For this review, use the dimensioned drawing (mm, ordinates from the lowest corner) and the shaded views. Round coordinates to 2 decimals unless told otherwise and drop trailing zeros. Write each loop counter-clockwise with the first axis right and the second up, starting at its lowest first coordinate (ties: lowest second). Pieces come first, ordered by that corner, then holes. Notation, with made-up numbers: M -18,73 L 29,73 A16 ccw 29,85 Z; hole C 61.25,-37.5 d5. An arc over 180 degrees is marked long. Use one line per item in the form item = value. Start each with the question number.
Item 1: Add section B-B (z = 16.75). State the section outline as (x, y) points, and give its area (3 significant figures).
Item 2: Add section A-A (x = 71). State the section outline as (y, z) points, and give its area (3 significant figures).
Item 3: For line 1 (Y direction, x = 20, z = 11); line 2 (X direction, y = 615, z = 21.5); line 3 (Y direction, x = 26, z = 9.5), list the stretches that pass through material, from the lowest coordinate up. Write a range as [from, to].
Item 4: For P1, Ø8, axis at x = 49.5, z = 4, coming from the -Y side; P2, Ø3, axis at x = 64, z = 12, coming from the -Y side; P3, Ø2, axis at x = 8, z = 8, coming from the -Y side, all flat-tipped, find the tip position at first contact; note any pin that passes through.
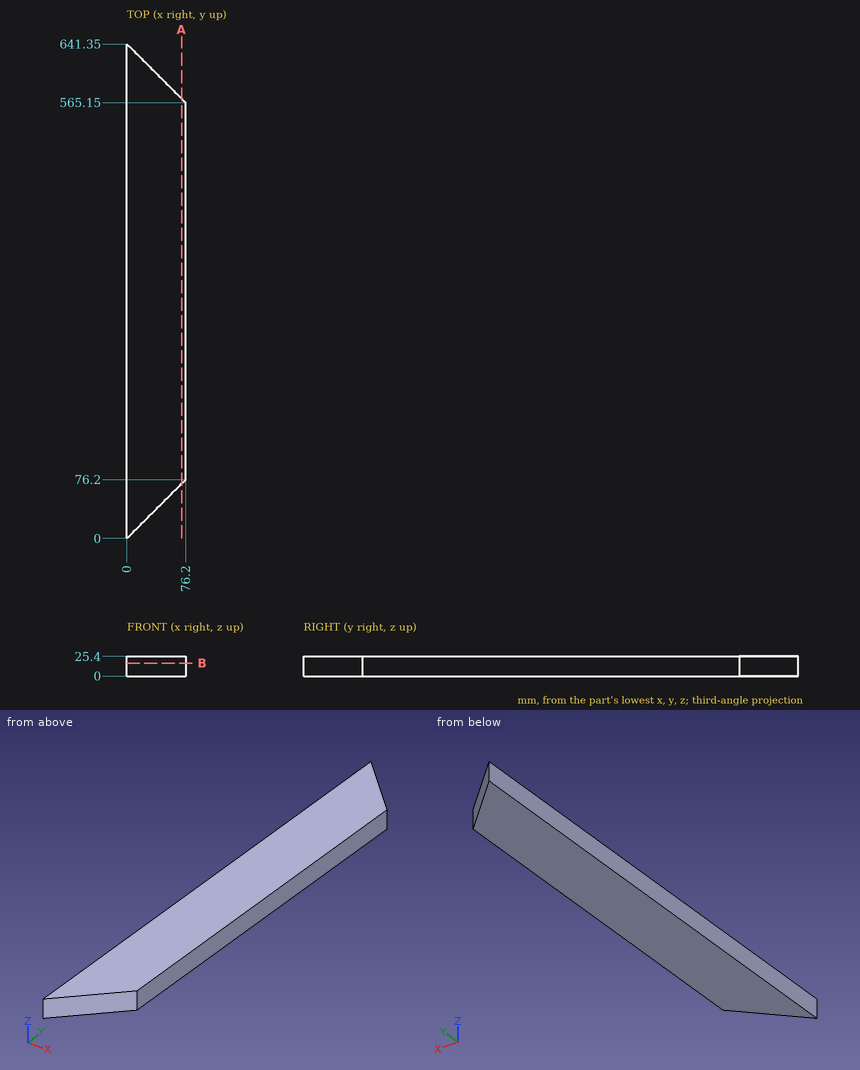
Calculated:
q1.outline = M 0,0 L 76.2,76.2 L 76.2,565.15 L 0,641.35 Z
q1.area = 43,100 mm^2
q2.outline = M 71,0 L 570.35,0 L 570.35,25.4 L 71,25.4 Z
q2.area = 12,700 mm^2
q3.line_1 = [20, 621.35]
q3.line_2 = [0, 26.35]
q3.line_3 = [26, 615.35]
q4.P1 = 45.5
q4.P2 = 62.5
q4.P3 = 7
